```python
from build123d import *

# Parameters (mm, degrees)
SKETCH_1_W                = 160
SKETCH_1_H                = 80
EXTRUDE_1_DEPTH           = 80
SKETCH_10_W               = 21.5
SKETCH_10_H               = 15
CUT_EXTRUDE_6_DEPTH       = 10
SKETCH_11_W               = 55
SKETCH_11_H               = 80
CUT_EXTRUDE_7_DEPTH       = 38
SKETCH_12_W               = 55
SKETCH_12_H               = 80
CUT_EXTRUDE_8_DEPTH       = 38
SKETCH_14_W               = 95
SKETCH_14_H               = 70
CUT_EXTRUDE_9_DEPTH       = 75
SKETCH_15_W               = 102.8
SKETCH_15_H               = 77.8
SKETCH_15_W_2             = 97.2
SKETCH_15_H_2             = 72.2
CUT_EXTRUDE_10_DEPTH      = 10
SKETCH_16_W               = 5
SKETCH_16_H               = 5
SKETCH_16_R               = 1.1
EXTRUDE_2_DEPTH           = 5
SKETCH_17_R               = 5
CUT_EXTRUDE_12_DEPTH      = 9.2
SKETCH_18_W               = 23.5
SKETCH_18_H               = 13
CUT_EXTRUDE_13_DEPTH      = 9.2
SKETCH_19_W               = 5
SKETCH_19_H               = 5
SKETCH_19_R               = 1.1
EXTRUDE_3_DEPTH           = 12
SKETCH_20_R               = 1.1
CUT_EXTRUDE_14_DEPTH      = 5
CUT_EXTRUDE_14_DEPTH_BACK = 5


with BuildPart() as part:
    # 草圖1 → 填料-伸長1 (new body)
    with BuildSketch(Plane.XY):
        with Locations((4.491097826, 5.58988764)):
            Rectangle(SKETCH_1_W, SKETCH_1_H)
    extrude(amount=EXTRUDE_1_DEPTH)

    # 草圖10 → 除料-伸長6 (cut)
    with BuildSketch(Plane(origin=(0, -34.41011236, 0), x_dir=(-1, 0, 0), z_dir=(0, -1, 0))):
        with Locations((24.758902174, -22.5)):
            Rectangle(SKETCH_10_W, SKETCH_10_H)
    extrude(amount=-CUT_EXTRUDE_6_DEPTH, mode=Mode.SUBTRACT)

    # 草圖11 → 除料-伸長7 (cut)
    with BuildSketch(Plane(origin=(0, 0, 0), x_dir=(-1, 0, 0), z_dir=(0, 0, -1))):
        with Locations((-56.991097826, 5.58988764)):
            Rectangle(SKETCH_11_W, SKETCH_11_H)
    extrude(amount=-CUT_EXTRUDE_7_DEPTH, mode=Mode.SUBTRACT)

    # 草圖12 → 除料-伸長8 (cut)
    with BuildSketch(Plane.XY.offset(80)):
        with Locations((56.991097826, 5.58988764)):
            Rectangle(SKETCH_12_W, SKETCH_12_H)
    extrude(amount=-CUT_EXTRUDE_8_DEPTH, mode=Mode.SUBTRACT)

    # 草圖14 → 除料-伸長9 (cut)
    with BuildSketch(Plane(origin=(0, 0, 0), x_dir=(-1, 0, 0), z_dir=(0, 0, -1))):
        with Locations((23.008902174, 5.58988764)):
            Rectangle(SKETCH_14_W, SKETCH_14_H)
    extrude(amount=-CUT_EXTRUDE_9_DEPTH, mode=Mode.SUBTRACT)

    # 草圖15 → 除料-伸長10 (cut)
    with BuildSketch(Plane(origin=(0, 0, 0), x_dir=(-1, 0, 0), z_dir=(0, 0, -1))):
        with Locations((23.008902174, 5.58988764)):
            Rectangle(SKETCH_15_W, SKETCH_15_H)
        with Locations((23.008902174, 5.58988764)):
            Rectangle(SKETCH_15_W_2, SKETCH_15_H_2, mode=Mode.SUBTRACT)
    extrude(amount=-CUT_EXTRUDE_10_DEPTH, mode=Mode.SUBTRACT)

    # 草圖16 → 填料-伸長2 (add)
    with BuildSketch(Plane(origin=(0, 0, 0), x_dir=(-1, 0, 0), z_dir=(0, 0, -1))):
        with Locations((-26.991097826, 48.08988764)):
            Rectangle(SKETCH_16_W, SKETCH_16_H)
        with Locations((-26.991097826, 48.08988764)):
            Circle(SKETCH_16_R, mode=Mode.SUBTRACT)
        with Locations((73.008902174, 48.08988764)):
            Rectangle(SKETCH_16_W, SKETCH_16_H)
        with Locations((73.008902174, 48.08988764)):
            Circle(SKETCH_16_R, mode=Mode.SUBTRACT)
        with Locations((73.008902174, -36.91011236)):
            Rectangle(SKETCH_16_W, SKETCH_16_H)
        with Locations((73.008902174, -36.91011236)):
            Circle(SKETCH_16_R, mode=Mode.SUBTRACT)
        with Locations((-26.991097826, -36.91011236)):
            Rectangle(SKETCH_16_W, SKETCH_16_H)
        with Locations((-26.991097826, -36.91011236)):
            Circle(SKETCH_16_R, mode=Mode.SUBTRACT)
    extrude(amount=-EXTRUDE_2_DEPTH)

    # 草圖17 → 除料-伸長12 (cut)
    with BuildSketch(Plane(origin=(29.491097826, 0, 0), x_dir=(0, 0, -1), z_dir=(1, 0, 0))):
        with Locations((-63.691723703, 5.58988764)):
            Circle(SKETCH_17_R)
        with Locations((-16.308276297, 5.58988764)):
            Circle(SKETCH_17_R)
    extrude(amount=-CUT_EXTRUDE_12_DEPTH, mode=Mode.SUBTRACT)

    # 草圖18 → 除料-伸長13 (cut)
    with BuildSketch(Plane(origin=(0, 0, 38), x_dir=(-1, 0, 0), z_dir=(0, 0, -1))):
        with Locations((-65.741097826, 5.58988764)):
            Rectangle(SKETCH_18_W, SKETCH_18_H)
    extrude(amount=-CUT_EXTRUDE_13_DEPTH, mode=Mode.SUBTRACT)

    # 草圖19 → 填料-伸長3 (add)
    with BuildSketch(Plane(origin=(0, 0, 38), x_dir=(-1, 0, 0), z_dir=(0, 0, -1))):
        with Locations((-79.991097826, 5.58988764)):
            Rectangle(SKETCH_19_W, SKETCH_19_H)
        with Locations((-79.991097826, 5.58988764)):
            Circle(SKETCH_19_R, mode=Mode.SUBTRACT)
        with Locations((-51.491097826, 5.58988764)):
            Rectangle(SKETCH_19_W, SKETCH_19_H)
        with Locations((-51.491097826, 5.58988764)):
            Circle(SKETCH_19_R, mode=Mode.SUBTRACT)
    extrude(amount=-EXTRUDE_3_DEPTH)

    # 草圖20 → 除料-伸長14 (cut, two sides)
    with BuildSketch(Plane(origin=(0, 0, 38), x_dir=(-1, 0, 0), z_dir=(0, 0, -1))) as cut_extrude_14_sk:
        with Locations((-79.991097826, 5.58988764)):
            Circle(SKETCH_20_R)
        with Locations((-51.491097826, 5.58988764)):
            Circle(SKETCH_20_R)
    extrude(amount=CUT_EXTRUDE_14_DEPTH, mode=Mode.SUBTRACT)
    extrude(cut_extrude_14_sk.sketch, amount=-CUT_EXTRUDE_14_DEPTH_BACK, mode=Mode.SUBTRACT)


solid = part.part
```
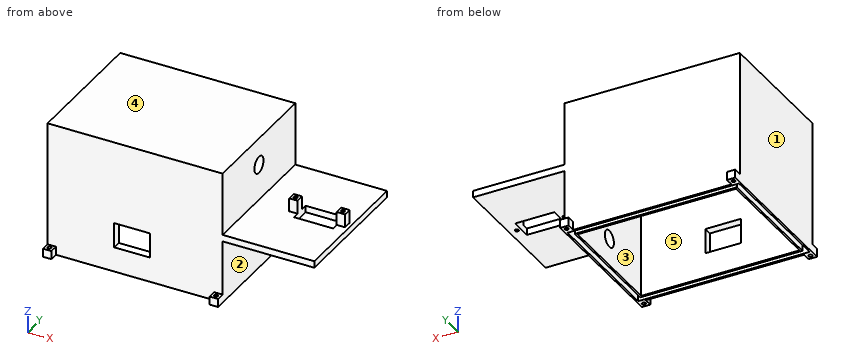
Here's how the part is built. I have some questions about the finished solid (model axes, mm). Face numbers are marked on the shaded views. A direction names the side the tool comes from. Coordinates: 2 decimals unless noted, no trailing zeros. Write each loop counter-clockwise with the first axis right and the second up, starting at its lowest first coordinate (ties: lowest second). Pieces come first, ordered by that corner, then holes. Notation, with made-up numbers: (78, 78) -> (104, 78) arc R16 ccw to (104, 93) -> close; hole circle Ø2 at (62.25, 65). An arc over 180 degrees is marked (long way). Use a Markdown table: item, result. Add a question column.
(1) If we section it at B-B, the plane z = 46.5: Write out the boundary of the cut face in (x, y), and give its area (3 significant figures).
(2) I'm going to push flat-ended pins straight in: P1, Ø5.5, axis at y = -36, z = 1.5, coming from the +X side; P2, Ø4, axis at x = 81, z = 47, coming from the -Y side; P3, Ø2, axis at x = 62.5, z = 40, coming from the +Y side. Where does each tip first touch, or does it pass through?
(3) We'd pull the mould along Y, two halves only. Please class the marked faces 4 and 5: +Y half, -Y half, draft (parallel to the pull), parting line (faces both ways), or undercut.
(4) If we section it at C-C, the plane z = 32.5: Write out the boundary of the cut face in (x, y), and give its area (3 significant figures).
(5) For the marked faces 1, 2 and 3, which set-ups out of +Z, -Z, +X, -X, +Y, -Y let a thin tool reach every point of the face, with its end or its side?
(6) Please list where these lines run through material, in increasing order: line 1 (Y direction, x = 11, z = 63.5); line 2 (X direction, y = 20.5, z = 58.5); line 3 (Z direction, x = 21, y = -14).
(7) If we section it at A-A, the plane x = 68: Write out the boundary of the cut face in (y, z), and give its area (3 significant figures).
(8) If we section it at D-D, the plane x = -6: Write out the boundary of the cut face in (y, z), and give its area (3 significant figures).
Outcome:
| question | item | result |
|---|---|---|
| 1 | outline | (-75.51, -34.41) -> (29.49, -34.41) -> (29.49, 45.59) -> (-75.51, 45.59) -> close; (48.99, 3.09) -> (53.99, 3.09) -> (53.99, 8.09) -> (48.99, 8.09) -> close; (77.49, 3.09) -> (82.49, 3.09) -> (82.49, 8.09) -> (77.49, 8.09) -> close; hole (-70.51, -29.41) -> (24.49, -29.41) -> (24.49, 40.59) -> (-70.51, 40.59) -> close; hole circle Ø2.2 at (51.49, 5.59); hole circle Ø2.2 at (79.99, 5.59) |
| 1 | area | 1,790 mm^2 |
| 2 | P1 | stops at x = 29.49 |
| 2 | P2 | stops at y = 3.09 |
| 2 | P3 | stops at y = 45.59 |
| 3 | face 4 | draft |
| 3 | face 5 | undercut |
| 4 | outline | (-75.51, -34.41) -> (29.49, -34.41) -> (29.49, 45.59) -> (-75.51, 45.59) -> close; hole (-70.51, -29.41) -> (24.49, -29.41) -> (24.49, 40.59) -> (-70.51, 40.59) -> close |
| 4 | area | 1,750 mm^2 |
| 5 | face 1 | +Z, -Z, -X, +Y, -Y |
| 5 | face 2 | -Z, +X, +Y, -Y |
| 5 | face 3 | -Z |
| 6 | line 1 | y = -34.41 to -29.41, 40.59 to 45.59 |
| 6 | line 2 | x = -75.51 to -70.51, 24.49 to 29.49 |
| 6 | line 3 | z = 75 to 80 |
| 7 | outline | (-34.41, 38) -> (-0.91, 38) -> (-0.91, 42) -> (-34.41, 42) -> close; (12.09, 38) -> (45.59, 38) -> (45.59, 42) -> (12.09, 42) -> close |
| 7 | area | 268 mm^2 |
| 8 | outline | (-34.41, 0) -> (-33.31, 0) -> (-33.31, 10) -> (-30.51, 10) -> (-30.51, 0) -> (-29.41, 0) -> (-29.41, 75) -> (40.59, 75) -> (40.59, 0) -> (41.69, 0) -> (41.69, 10) -> (44.49, 10) -> (44.49, 0) -> (45.59, 0) -> (45.59, 80) -> (-34.41, 80) -> close |
| 8 | area | 1,090 mm^2 |
